Can you work these out from the model? Positions are in its coordinate system, mm. A direction names the side the tool comes from. Coordinates: 2 decimals unless noted, no trailing zeros. Write each loop counter-clockwise with the first axis right and the second up, starting at its lowest first coordinate (ties: lowest second). Pieces come first, ordered by that corner, then holes. Notation, with made-up numbers: (0.25, 78.5) - (57.25, 78.5) arc R10 ccw to (57.25, 97.5) - close; hole circle Ø2 at (16.25, 25). An arc over 180 degrees is marked (long way). Use one line per item in the form item = value. Start each with the question number.
(1) If we section it at D-D on y = -16.5: Please give me the cut outline in (x, z).
(2) If I drill on probe 1 along Y at (x, z) = (55, 17.5); probe 2 along X at (y, z) = (67.5, 20.5); probe 3 along Y at (x, z) = (19, 35), over which ranges is the centre line in solid material (lowest first)? Write a range as from..to.
(3) Thinking about a two-plate mould opening in X: for faces 1 (the face through (60, -1, 22)), 2 (the face through (-1, -72.5, 22)), 3 (the face through (-1, 70, 23)), which applies, pulls with the +X half, pulls with the -X half, needs draft (parallel to the pull), parting line crosses it, or undercut?
(4) On a 3-axis mill with a long thin cutter (end or side, diameter ignored), from which of +Z, -Z, +X, -X, +Y, -Y can I reach the whole of each face in a straight line? I mean faces 4 (the face through (-1, 1, 0)), 5 (the face through (-57.5, -1, 23)). Say none if no direction works.
(5) For pin 1 Ø1.8 at (x, y) = (55, -67.5) entering from +Z; pin 2 Ø5 at (x, y) = (-45, -1.5) entering from +Z, each with a flat end and sliding along its axis, tell me the tip position at first contact or that it passes through.
(6) If we section it at A-A on y = -41.5: Please give me the cut outline in (x, z), then the cut area to 3 significant figures.
(7) If we section it at C-C on z = 36: Please give me the cut outline in (x, y), then the cut area to 3 significant figures.
(8) If we section it at B-B on x = 33: Please give me the cut outline in (y, z).
```python
from build123d import *

# Parameters (mm, degrees)
F4_W      = 120
F4_H      = 145
F5_DEPTH  = 45
F6_T      = -2.5
F8_W      = 35
F8_H      = 45
F8_W_2    = 21.5
F8_H_2    = 29.6
F7_W      = 84.7
F7_H      = 44.7
F9_DEPTH  = 2.5
F10_W     = 5
F10_H     = 5
F11_DEPTH = 42.5
F12_R     = 1.15
F13_DEPTH = 36
F14_R     = 2.3


with BuildPart() as f5:
    # F4 (on Top) → F5 (new body)
    with BuildSketch(Plane.XY):
        Rectangle(F4_W, F4_H)
    extrude(amount=F5_DEPTH)

    # F6
    f6_openings = [f5.faces().sort_by_distance(p)[0] for p in [
        (0, 0, 45),
    ]]
    offset(amount=F6_T, openings=f6_openings)

    # F8 (on face) + F7 (on face) → F9 (cut)
    with BuildSketch(Plane.XY.offset(2.5)):
        with Locations((-18, -27.2)):
            Rectangle(F8_W, F8_H)
        with Locations((32.25, -21.4211801112)):
            Rectangle(F8_W_2, F8_H_2)
    with BuildSketch(Plane.XY.offset(2.5)):
        with Locations((0, 32.65)):
            Rectangle(F7_W, F7_H)
    extrude(amount=-F9_DEPTH, mode=Mode.SUBTRACT)

    # F10 (on face) → F11 (join)
    with BuildSketch(Plane.XY.offset(2.5)):
        with Locations((-55, 67.5)):
            Rectangle(F10_W, F10_H)
        with Locations((-55, -67.5)):
            Rectangle(F10_W, F10_H)
        with Locations((55, -67.5)):
            Rectangle(F10_W, F10_H)
        with Locations((55, 67.5)):
            Rectangle(F10_W, F10_H)
    extrude(amount=F11_DEPTH)

    # F12 (on face) → F13 (cut)
    with BuildSketch(Plane.XY.offset(45)):
        with Locations((-55, 67.5)):
            Circle(F12_R)
        with Locations((55, 67.5)):
            Circle(F12_R)
        with Locations((55, -67.5)):
            Circle(F12_R)
        with Locations((-55, -67.5)):
            Circle(F12_R)
    extrude(amount=-F13_DEPTH, mode=Mode.SUBTRACT)

    # F14
    f14_edges = [f5.edges().sort_by_distance(p)[0] for p in [
        (-52.5, 65, 23.75),
        (52.5, 65, 23.75),
        (52.5, -65, 23.75),
        (-52.5, -65, 23.75),
    ]]
    fillet(f14_edges, radius=F14_R)


solid = f5.part
```
Reported:
q1.outline = (-60, 0) - (-35.5, 0) - (-35.5, 2.5) - (-57.5, 2.5) - (-57.5, 45) - (-60, 45) - close; (-0.5, 0) - (21.5, 0) - (21.5, 2.5) - (-0.5, 2.5) - close; (43, 0) - (60, 0) - (60, 45) - (57.5, 45) - (57.5, 2.5) - (43, 2.5) - close
q2.probe_1 = -72.5..-68.65, -66.35..-65, 65..66.35, 68.65..72.5
q2.probe_2 = -60..-56.15, -53.85..-52.5, 52.5..53.85, 56.15..60
q2.probe_3 = -72.5..-70, 70..72.5
q3.face_1 = pulls with the +X half
q3.face_2 = needs draft
q3.face_3 = undercut
q4.face_4 = -Z, +X, -X, +Y, -Y
q4.face_5 = +Z
q5.pin_1 = 9
q5.pin_2 = 2.5
q6.outline = (-60, 0) - (-35.5, 0) - (-35.5, 2.5) - (-57.5, 2.5) - (-57.5, 45) - (-60, 45) - close; (-0.5, 0) - (60, 0) - (60, 45) - (57.5, 45) - (57.5, 2.5) - (-0.5, 2.5) - close
q6.area = 425 mm2
q7.outline = (-60, -72.5) - (60, -72.5) - (60, 72.5) - (-60, 72.5) - close; hole (-57.5, -65) - (-54.8, -65) arc R2.3 cw to (-52.5, -67.3) - (-52.5, -70) - (52.5, -70) - (52.5, -67.3) arc R2.3 cw to (54.8, -65) - (57.5, -65) - (57.5, 65) - (54.8, 65) arc R2.3 cw to (52.5, 67.3) - (52.5, 70) - (-52.5, 70) - (-52.5, 67.3) arc R2.3 cw to (-54.8, 65) - (-57.5, 65) - close; hole circle Ø2.3 at (-55, -67.5); hole circle Ø2.3 at (-55, 67.5); hole circle Ø2.3 at (55, -67.5); hole circle Ø2.3 at (55, 67.5)
q7.area = 1,380 mm2
q8.outline = (-72.5, 0) - (-36.22, 0) - (-36.22, 2.5) - (-70, 2.5) - (-70, 45) - (-72.5, 45) - close; (-6.62, 0) - (10.3, 0) - (10.3, 2.5) - (-6.62, 2.5) - close; (55, 0) - (72.5, 0) - (72.5, 45) - (70, 45) - (70, 2.5) - (55, 2.5) - close
